from build123d import *

# Parameters (mm, degrees)
SKETCH_2_R         = 7.5
EXTRUDE_1_DEPTH    = 5
HOLE_WIZARD_M4_1_D = 3.3


with BuildPart() as part:
    # 草圖2 → 填料-伸長1 (new body, symmetric)
    with BuildSketch(Plane(origin=(0, 0, 0), x_dir=(1, 0, 0), z_dir=(0, 1, 0))):
        Polygon((-12.5, -40), (-12.5, -15), (-30, -15), (-30, 0), (30, 0), (30, -15), (12.5, -15), (12.5, -40), align=None)
        with Locations((0, -27.5)):
            Circle(SKETCH_2_R, mode=Mode.SUBTRACT)
    extrude(amount=EXTRUDE_1_DEPTH, both=True)

    # M4 螺紋孔1 (through all)
    with Locations(Plane(origin=(0, 0, 0), x_dir=(-1, 0, 0), z_dir=(0, 0, -1))):
        with Locations((-23.75, 0), (23.75, 0)):
            Hole(HOLE_WIZARD_M4_1_D / 2)


solid = part.part
CAD build for the part. Positions are in the model's coordinates, mm. A direction names the side the tool comes from. Round coordinates to 2 decimals unless told otherwise and drop trailing zeros. Loops run counter-clockwise (first coordinate to the right, second up) from the corner with the lowest first, then second, coordinate; pieces in that order, holes last. Notation, with made-up numbers: (-9, 81) - (8, 81) arc R17 ccw to (8, 92) - close; hole circle Ø10 at (70, 52). An arc over 180 degrees is marked (long way). Put each result on its own line as item: value.
1. Two-plate mould, pull along X, no slides. Class faces 4 (the flat face through (0, 0, 40)), 5 (the cylindrical face through (-25.4, 0.07, 7.61)), 6 (the flat face through (-12.5, 0, 28)): released by +X, released by -X, zero draft, split by the parting line, or undercut.
Geometry check:
face 4: zero draft
face 5: undercut
face 6: released by -X
2. Slice it at B-B on y = -2.75. List the corners of the cut face in (x, z).
Geometry check:
outline: (-30, 0) - (30, 0) - (30, 15) - (12.5, 15) - (12.5, 40) - (-12.5, 40) - (-12.5, 15) - (-30, 15) - close; hole circle Ø15 at (0, 27.5)
3. Slice it at A-A on x = 23.75. List the corners of the cut face in (y, z).
Geometry check:
outline: (-5, 0) - (-1.65, 0) - (-1.65, 15) - (-5, 15) - close; (1.65, 0) - (5, 0) - (5, 15) - (1.65, 15) - close
4. Wall check: line 1 (X direction, y = 2.75, z = 27.5); line 2 (Y direction, x = 23.75, z = 4); line 3 (Z direction, x = 0, y = 1.75). Give the ranges that are in metal, low to high.
Geometry check:
line 1: -12.5 to -7.5, 7.5 to 12.5
line 2: -5 to -1.65, 1.65 to 5
line 3: 0 to 20, 35 to 40
5. Slice it at C-C on z = 27.5. List the corners of the cut face in (x, y).
Geometry check:
outline: (-12.5, -5) - (-7.5, -5) - (-7.5, 5) - (-12.5, 5) - close; (7.5, -5) - (12.5, -5) - (12.5, 5) - (7.5, 5) - close
6. Slice it at D-D on x = 15.5. List the corners of the cut face in (y, z), and give its area (3 significant figures).
Geometry check:
outline: (-5, 0) - (5, 0) - (5, 15) - (-5, 15) - close
area: 150 mm²
7. 3-axis set-ups, long thin cutter, end or side, ignore diameter. For faces 1 (the cylindrical face through (22.1, 0.07, 7.61)), 2 (the flat face through (-21, 0, 15)), 3 (the flat face through (21, 0, 15)): which of +Z, -Z, +X, -X, +Y, -Y reach the whole face in a straight line?
Geometry check:
face 1: +Z, -Z
face 2: +Z, -X, +Y, -Y
face 3: +Z, +X, +Y, -Y
8. Pin check, flat tips, straight feed: P1, Ø3, axis at y = -1, z = 23.5, coming from the +X side; P2, Ø5, axis at y = 1, z = 33, coming from the -X side; P3, Ø5.5, axis at x = -23.75, y = 0, coming from the -Z side. Stop position of each tip, or through.
Geometry check:
P1: x = 12.5
P2: x = -12.5
P3: z = 0
